The listing builds one solid part. Answer for the finished solid, in the listing's coordinates (mm). Face numbers are marked on the shaded views. A direction names the side the tool comes from. Round coordinates to 2 decimals unless told otherwise and drop trailing zeros. Write each loop counter-clockwise with the first axis right and the second up, starting at its lowest first coordinate (ties: lowest second). Pieces come first, ordered by that corner, then holes.
Item 1: Each of these flat-tipped pins is pushed along its axis until it touches: pin 1 (4 mm diameter, centred on y = -21, z = -10, fed in from +X); pin 2 (4 mm diameter, centred on x = -17, y = -14.5, fed in from -Z) (3 decimals); pin 3 (1.9 mm diameter, centred on x = 44.81, z = 8.45, fed in from +Y); pin 4 (3 mm diameter, centred on y = -39, z = 1.5, fed in from -X). Where does it stop, or does it pass through?
Item 2: For a pull along X with two mould halves and no side action, classify the marked faces 1, 2 and 3 as +X half, -X half, draft (parallel to the pull), parting line (faces both ways), or undercut.
Item 3: Find section A-A on x = 0. Give the vertices of the cut face in (y, z) (3 decimals), then the cut area to 3 significant figures.
Item 4: Find the intervals of material crossed by probe 1 along X at (y, z) = (-29.55, 1.25); probe 2 along X at (y, z) = (-34, -10.5); probe 3 along Y at (x, z) = (61.5, -10), in increasing order.
Item 5: Find section B-B on y = -21. Give the vertices of the cut face in (x, z) (3 decimals).
Item 6: Find section C-C on y = -29.55. Give the vertices of the cut face in (x, z) (3 decimals).
Item 7: A tool of negligible diameter and unlimited length cuts with its end or side. For the marked faces 4, 5 and 6, from which of +Z, -Z, +X, -X, +Y, -Y can it reach the whole face along a straight path? Write none if from no direction.
Item 8: Find section D-D on x = -42. Give the vertices of the cut face in (y, z) (3 decimals), then the cut area to 3 significant figures.
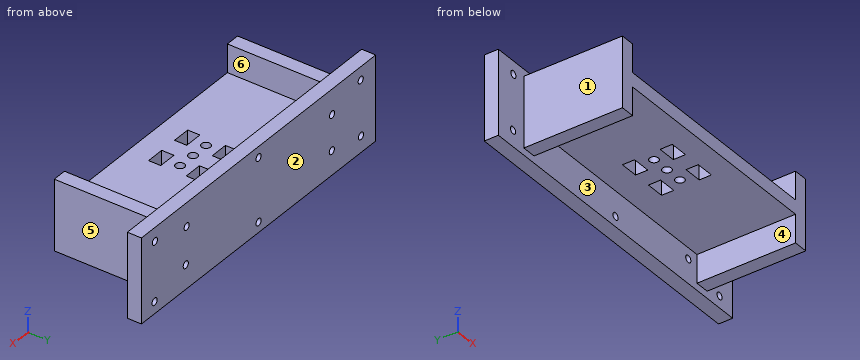
```python
from build123d import *

# Parameters (mm, degrees)
F0_W      = 146.05
F0_H      = 38.1
F1_DEPTH  = 6.35
F2_W      = 101.6
F2_H      = 6.35
F3_DEPTH  = 44.45
F4_W      = 6.35
F4_H      = 31.75
F5_DEPTH  = 44.45
F6_R      = 1.6
F7_DEPTH  = 6.351
F8_W      = 8.2
F8_H      = 5.5
F9_DEPTH  = 22.226
F10_R     = 2
F11_DEPTH = 22.226


with BuildPart() as f1:
    # F0 (on Front) → F1 (new body)
    with BuildSketch(Plane.XZ):
        Rectangle(F0_W, F0_H)
    extrude(amount=F1_DEPTH)

    # F2 (on face) → F3 (join)
    with BuildSketch(Plane.XZ.offset(6.35)):
        Rectangle(F2_W, F2_H)
    extrude(amount=F3_DEPTH)

    # F4 (on face) → F5 (join)
    with BuildSketch(Plane.XZ.offset(6.35)):
        with Locations((-53.957961, 0)):
            Rectangle(F4_W, F4_H)
        with Locations((53.957961, 0)):
            Rectangle(F4_W, F4_H)
    extrude(amount=F5_DEPTH)

    # F6 (on face) → F7 (cut, through all)
    with BuildSketch(Plane.XZ.offset(6.35)):
        with Locations((0, 14.169781)):
            Circle(F6_R)
        with Locations((44.810925, 8.448409)):
            Circle(F6_R)
        with Locations((64.655818, 12.911452)):
            Circle(F6_R)
        with Locations((64.852946, -13.699939)):
            Circle(F6_R)
        with Locations((45.368467, -8.138511)):
            Circle(F6_R)
        with Locations((0, -14.424114)):
            Circle(F6_R)
        with Locations((-45.650516, -8.138511)):
            Circle(F6_R)
        with Locations((-45.789901, 7.751479)):
            Circle(F6_R)
        with Locations((-63.670218, 13.108574)):
            Circle(F6_R)
        with Locations((-63.867338, -11.728724)):
            Circle(F6_R)
    extrude(amount=-F7_DEPTH, mode=Mode.SUBTRACT)

    # F8 (on face) → F9 (cut, through all)
    with BuildSketch(Plane(origin=(0, 0, -3.175), x_dir=(1, 0, 0), z_dir=(0, 0, -1))):
        with Locations((-8.117039, 38.05)):
            Rectangle(F8_W, F8_H)
        with Locations((8.082961, 38.05)):
            Rectangle(F8_W, F8_H)
        with Locations((-8.117039, 21.05)):
            Rectangle(F8_W, F8_H)
        with Locations((8.082961, 21.05)):
            Rectangle(F8_W, F8_H)
    extrude(amount=-F9_DEPTH, mode=Mode.SUBTRACT)

    # F10 (on face) → F11 (cut, through all)
    with BuildSketch(Plane(origin=(0, 0, -3.175), x_dir=(1, 0, 0), z_dir=(0, 0, -1))):
        with Locations((0, 29.55)):
            Circle(F10_R)
        with Locations((8.083, 29.55)):
            Circle(F10_R)
        with Locations((-8.083, 29.55)):
            Circle(F10_R)
    extrude(amount=-F11_DEPTH, mode=Mode.SUBTRACT)


solid = f1.part
```
Check values:
1. pin 1: stops at x = 57.13
1. pin 2: stops at z = -3.175
1. pin 3: passes through
1. pin 4: stops at x = -57.13
2. face 1: -X half
2. face 2: draft
2. face 3: undercut
3. outline: (-50.8, -3.175) - (-31.55, -3.175) - (-31.55, 3.175) - (-50.8, 3.175) - close; (-27.55, -3.175) - (-6.35, -3.175) - (-6.35, -12.824) - (0, -12.824) - (0, 12.57) - (-6.35, 12.57) - (-6.35, 3.175) - (-27.55, 3.175) - close; (-6.35, -19.05) - (0, -19.05) - (0, -16.024) - (-6.35, -16.024) - close; (-6.35, 15.77) - (0, 15.77) - (0, 19.05) - (-6.35, 19.05) - close
3. area: 458 mm2
4. probe 1: x = -57.13 to -10.08, -6.08 to -2, 2 to 6.08, 10.08 to 57.13
4. probe 2: x = -57.13 to -50.78, 50.78 to 57.13
4. probe 3: y = -6.35 to 0
5. outline: (-57.133, -15.875) - (-50.783, -15.875) - (-50.783, -3.175) - (-12.217, -3.175) - (-12.217, 3.175) - (-50.783, 3.175) - (-50.783, 15.875) - (-57.133, 15.875) - close; (-4.017, -3.175) - (3.983, -3.175) - (3.983, 3.175) - (-4.017, 3.175) - close; (12.183, -3.175) - (50.783, -3.175) - (50.783, -15.875) - (57.133, -15.875) - (57.133, 15.875) - (50.783, 15.875) - (50.783, 3.175) - (12.183, 3.175) - close
6. outline: (-57.133, -15.875) - (-50.783, -15.875) - (-50.783, -3.175) - (-10.083, -3.175) - (-10.083, 3.175) - (-50.783, 3.175) - (-50.783, 15.875) - (-57.133, 15.875) - close; (-6.083, -3.175) - (-2, -3.175) - (-2, 3.175) - (-6.083, 3.175) - close; (2, -3.175) - (6.083, -3.175) - (6.083, 3.175) - (2, 3.175) - close; (10.083, -3.175) - (50.783, -3.175) - (50.783, -15.875) - (57.133, -15.875) - (57.133, 15.875) - (50.783, 15.875) - (50.783, 3.175) - (10.083, 3.175) - close
7. face 4: -Z, -Y
7. face 5: +Z, -Z, +X, -Y
7. face 6: +Z, -Y
8. outline: (-50.8, -3.175) - (-6.35, -3.175) - (-6.35, -19.05) - (0, -19.05) - (0, 19.05) - (-6.35, 19.05) - (-6.35, 3.175) - (-50.8, 3.175) - close
8. area: 524 mm2
